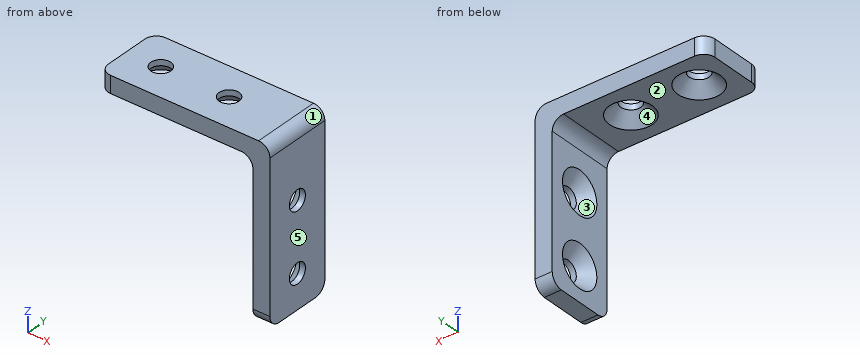
Autodesk Inventor part; units mm, degrees
ref_plane "YZ Plane" through (0, 0, 0) normal (1, 0, 0) x (0, 1, 0)
ref_plane "XZ Plane" through (0, 0, 0) normal (0, 1, 0) x (-1, 0, 0)
ref_plane "XY Plane" through (0, 0, 0) normal (0, 0, 1) x (1, 0, 0)
sketch "Sketch1" plane through (0, 0, 0) normal (0, 1, 0) x (-1, 0, 0)
  line L0 (0, 0) -> (30, 0)
  line L1 (30, 0) -> (30, -3)
  line L2 (30, -3) -> (3, -3)
  line L3 (3, -3) -> (3, -30)
  line L4 (3, -30) -> (0, -30)
  line L5 (0, -30) -> (0, 0)
  dimension "d0" = 3
  dimension "d1" = 3
  dimension "d4" = 30
  dimension "d5" = 30
extrude "Extrusion1" add sketch "Sketch1" along normal blind 12
sketch "Sketch2" plane through (-3, 0, -30) normal (-1, 0, 0) x (0, 0, 1)
  line L0 (0, 0) -> (0, 12)
  line L1 (0, 6) -> (27, 6) construction
  line L2 (27, 0) -> (27, 12)
  circle A0 centre (6, 6) radius 1.75
  circle A1 centre (18, 6) radius 1.75
  point P0 (30, 0)
  dimension "d8" = 3.5
  dimension "d9" = 3.5
  dimension "d10" = 6
  dimension "d11" = 12
extrude "Extrusion2" cut sketch "Sketch2" against normal blind 12
sketch "Sketch3" plane through (-3, 0, -3) normal (0, 0, -1) x (-1, 0, 0)
  line L0 (27, 0) -> (27, 12)
  line L1 (27, 6) -> (0, 6) construction
  line L2 (0, 0) -> (0, 12)
  circle A0 centre (21, 6) radius 1.75
  circle A1 centre (9, 6) radius 1.75
  point P0 (-3, 0)
  dimension "d14" = 6
  dimension "d15" = 12
  dimension "d16" = 3.5
  dimension "d17" = 3.5
extrude "Extrusion3" cut sketch "Sketch3" against normal blind 12
chamfer "Chamfer1" distance 2 angle 45 4 edges at (-22.25, 6, -3) (-10.25, 6, -3) (-3, 6, -13.75) (-3, 6, -25.75)
fillet "Fillet1" radius 2 6 edges at (-1.5, 12, -30) (-1.5, 0, -30) (-30, 12, -1.5) (-30, 0, -1.5) (-3, 6, -3) (0, 6, 0)
properties part number "Bracket"
Design review of the part built by this model. Coordinates are the model's own, in mm. Face numbers are marked on the shaded views. A direction names the side the tool comes from. Round coordinates to 2 decimals unless told otherwise and drop trailing zeros. Write each loop counter-clockwise with the first axis right and the second up, starting at its lowest first coordinate (ties: lowest second). Pieces come first, ordered by that corner, then holes. Notation, with made-up numbers: (57.5, -17) -> (110.5, -17) arc R36 cw to (110.5, 19) -> close; hole circle Ø2 at (-36.75, 10). An arc over 180 degrees is marked (long way). One line per question, with ' | ' between items.
(1) Machinability: for the marked faces 1 and 2, which of the approach directions +Z, -Z, +X, -X, +Y, -Y give a long, thin tool a straight path to every point of the face, cutting with its end or side? Answer none if there is none.
Result sheet:
face 1: +Z, +X, +Y, -Y | face 2: -Z, -X, +Y, -Y
(2) Take a section at D-D, the plane x = -19.5. State the section outline as (y, z) points.
Result sheet:
outline: (0, -3) -> (12, -3) -> (12, 0) -> (0, 0) -> close
(3) Take a section at B-B, the plane x = -24. State the section outline as (y, z) points, and give its area (3 significant figures).
Result sheet:
outline: (0, -3) -> (2.25, -3) -> (4.25, -1) -> (4.25, 0) -> (0, 0) -> close; (7.75, -1) -> (9.75, -3) -> (12, -3) -> (12, 0) -> (7.75, 0) -> close | area: 21.5 mm2
(4) Wall thickness on line 1 (Y direction, x = -0.4, z = -24); line 2 (Z direction, x = -10.25, y = 1.5): over which ranges is each line inside the solid? List them lowest first. Write a range as [from, to].
Result sheet:
line 1: [0, 4.25], [7.75, 12] | line 2: [-3, 0]
(5) Take a section at C-C, the plane y = 6. State how many separate pieces and enclosed holes the cut face has, and give its area (3 significant figures).
Result sheet:
separate pieces: 5 | enclosed holes: 0 | area: 113 mm2
(6) Insertion check: P1, Ø4, axis at y = 6, z = -18.5, coming from the -X side; P2, Ø1.5, axis at x = -20.5, y = 9, coming from the -Z side; P3, Ø3, axis at y = 6, z = -12, coming from the -X side; P4, Ø4.5, axis at x = -24, y = 6, coming from the -Z side. Each pin has a flat end and moves straight along its axis. Give the tip position at first contact, or say it passes through.
Result sheet:
P1: x = -3 | P2: z = -3 | P3: through | P4: z = -1.5
(7) Draft analysis for pull direction Z (two halves, no side actions). For the marked faces 3, 4 and 5, state which applies: released by +Z, released by -Z, zero draft, split by the parting line, or undercut.
Result sheet:
face 3: undercut | face 4: released by -Z | face 5: zero draft
(8) Take a section at A-A, the plane z = -12. State the section outline as (x, y) points.
Result sheet:
outline: (-3, 0) -> (0, 0) -> (0, 4.25) -> (-1, 4.25) -> (-3, 2.25) -> close; (-3, 9.75) -> (-1, 7.75) -> (0, 7.75) -> (0, 12) -> (-3, 12) -> close
